For this review, take the finished solid that the model builds, in its own axes (mm). Face numbers are marked on the shaded views. Give positions to 0.01 mm unless a question says otherwise; leave off trailing zeros. Write each loop counter-clockwise with the first axis right and the second up, starting at its lowest first coordinate (ties: lowest second). Pieces come first, ordered by that corner, then holes. Notation, with made-up numbers: (63, 32) -> (86, 32) arc R22 cw to (86, 65) -> close; hole circle Ø10 at (87, 28). An arc over 180 degrees is marked (long way). Return JSON: item names as keys, results as strings.
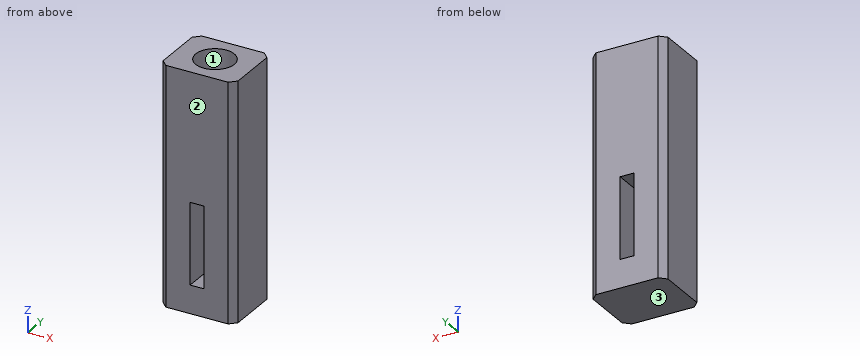
Autodesk Fusion 360 part; units mm, degrees
sketch "Sketch1" plane through (0, 0, 0) normal (0, 1, 0) x (1, 0, 0)
  line L0 (0.55, 3.25) -> (-0.55, 3.25)
  line L1 (-0.55, 3.25) -> (-0.55, -3.25)
  line L2 (-0.55, -3.25) -> (0.55, -3.25)
  line L3 (0.55, -3.25) -> (0.55, 3.25)
  line L4 (0.55, 3.25) -> (-0.55, -3.25) construction
  line L5 (-0.55, 3.25) -> (0.55, -3.25) construction
  line L6 (3, -5.5) -> (-3, -5.5)
  line L7 (-3, -5.5) -> (-3, 5.5)
  line L8 (-3, 5.5) -> (3, 5.5)
  line L9 (3, 5.5) -> (3, -5.5)
  line L10 (3, -5.5) -> (-3, 5.5) construction
  line L11 (-3, -5.5) -> (3, 5.5) construction
  dimension "d1" = 1.1
  dimension "d2" = 6.5
  dimension "d3" = 6
  dimension "d4" = 11
sketch "Sketch2" plane through (0, 0, 0) normal (0, 1, 0) x (1, 0, 0)
extrude "Extrude1" add sketch "Sketch1" along normal blind 5
extrude "Extrude2" add 1 faces at (1, 1.6667, 5.5) along direction (0, 0, 1) blind 8
hole "Hole1" at (0, 2.5, 13.5) direction (0, 0, -1) diameter 3.1 depth 9 tip angle 180
chamfer "Chamfer1" distance 0.5 angle 45 4 edges at (3, 5, 4) (-3, 5, 4) (3, 0, 4) (-3, 0, 4)
1. Add section C-C, the plane y = 2.5. State the section outline as (x, z) points, plus the area to 4 significant figures.
Results found:
{"outline": "(-3, -5.5) -> (3, -5.5) -> (3, 13.5) -> (1.55, 13.5) -> (1.55, 4.5) -> (-1.55, 4.5) -> (-1.55, 13.5) -> (-3, 13.5) -> close; hole (-0.55, -3.25) -> (0.55, -3.25) -> (0.55, 3.25) -> (-0.55, 3.25) -> close", "area": "78.95 mm²"}
2. For pin 1 (3 mm diameter, centred on x = 0.5, z = 2.5, fed in from +Y), flat-tipped, find the tip position at first contact; note if it passes through.
Results found:
{"pin 1": "stops at y = 5"}
3. To check wall thickness, follow probe 1 along X at (y, z) = (1.2, 2.75); probe 2 along Z at (x, y) = (-0.5, 0.85); probe 3 along X at (y, z) = (2.5, 10.75). State the ranges of each line that lie inside material, in increasing order.
Results found:
{"probe 1": "x = -3 to -0.55, 0.55 to 3", "probe 2": "z = -5.5 to -3.25, 3.25 to 13.5", "probe 3": "x = -3 to -1.55, 1.55 to 3"}
4. The part is to be moulded in two halves that separate along Y. For the marked faces 1, 2 and 3, say which applies: +Y half, -Y half, draft (parallel to the pull), parting line (faces both ways), or undercut.
Results found:
{"face 1": "undercut", "face 2": "-Y half", "face 3": "draft"}
5. Add section B-B, the plane x = 0. State the section outline as (y, z) points.
Results found:
{"outline": "(0, -5.5) -> (5, -5.5) -> (5, -3.25) -> (0, -3.25) -> close; (0, 3.25) -> (5, 3.25) -> (5, 13.5) -> (4.05, 13.5) -> (4.05, 4.5) -> (0.95, 4.5) -> (0.95, 13.5) -> (0, 13.5) -> close"}
6. Add section D-D, the plane z = 10. State the section outline as (x, y) points.
Results found:
{"outline": "(-3, 0.5) -> (-2.5, 0) -> (2.5, 0) -> (3, 0.5) -> (3, 4.5) -> (2.5, 5) -> (-2.5, 5) -> (-3, 4.5) -> close; hole circle Ø3.1 at (0, 2.5)"}
7. Add section A-A, the plane z = -0.25. State the section outline as (x, y) points.
Results found:
{"outline": "(-3, 0.5) -> (-2.5, 0) -> (-0.55, 0) -> (-0.55, 5) -> (-2.5, 5) -> (-3, 4.5) -> close; (0.55, 0) -> (2.5, 0) -> (3, 0.5) -> (3, 4.5) -> (2.5, 5) -> (0.55, 5) -> close"}
